from build123d import *

# Parameters (mm, degrees)
F3_DEPTH = 2.541


with BuildPart() as f1:
    # F0 (on Right) → F1 (revolve)
    with BuildSketch(Plane.YZ):
        with BuildLine():
            Line((16.51, 0), (19.05, 0))
            ThreePointArc((19.05, 0), (18.404048, 4.918689), (16.51, 9.50381))
            Line((16.51, 9.50381), (16.51, 0))
        make_face()
    revolve(axis=Axis((0, 17.78, 0), (0, -1, 0)))

    # F2 (on face) → F3 (cut, through all)
    with BuildSketch(Plane.XZ.offset(-16.51)):
        with BuildLine():
            Line((1.016, -4.826), (1.527208, -7.465389))
            ThreePointArc((1.527208, -7.465389), (5.388154, -5.388154), (7.465389, -1.527208))
            Line((7.465389, -1.527208), (4.826, -1.016))
            Line((4.826, -1.016), (4.826, 0))
            Line((4.826, 0), (4.826, 1.016))
            Line((4.826, 1.016), (7.465389, 1.527208))
            ThreePointArc((7.465389, 1.527208), (5.388154, 5.388154), (1.527208, 7.465389))
            Line((1.527208, 7.465389), (1.016, 4.826))
            Line((1.016, 4.826), (0, 4.826))
            Line((0, 4.826), (-1.016, 4.826))
            Line((-1.016, 4.826), (-1.527208, 7.465389))
            ThreePointArc((-1.527208, 7.465389), (-5.388154, 5.388154), (-7.465389, 1.527208))
            Line((-7.465389, 1.527208), (-4.826, 1.016))
            Line((-4.826, 1.016), (-4.826, 0))
            Line((-4.826, 0), (-4.826, -1.016))
            Line((-4.826, -1.016), (-7.465389, -1.527208))
            ThreePointArc((-7.465389, -1.527208), (-5.388154, -5.388154), (-1.527208, -7.465389))
            Line((-1.527208, -7.465389), (-1.016, -4.826))
            Line((-1.016, -4.826), (0, -4.826))
            Line((0, -4.826), (1.016, -4.826))
        make_face()
    extrude(amount=-F3_DEPTH, mode=Mode.SUBTRACT)


solid = f1.part
Part model, mm, in its own coordinate system. Coordinates: 2 decimals unless noted, no trailing zeros.
(1) Pull direction Z, two halves, no side cores. Call faces 1 (the face through (-0.7, 16.51, -5)), 2 (the face through (0, 17, 4.826)): pulls with the +Z half, pulls with the -Z half, needs draft (parallel to the pull), parting line crosses it, or undercut.
Check sheet entries:
face 1: needs draft
face 2: undercut
(2) Slice it at A-A, the plane x = 6.5. State how many separate pieces and enclosed holes the cut face has, and give its area (3 significant figures).
Check sheet entries:
separate pieces: 3
enclosed holes: 0
area: 6.79 mm2
(3) Pin check, flat tips, straight feed: pin 1 Ø0.6 at (y, z) = (17, 0.5) entering from +X; pin 2 Ø0.6 at (y, z) = (17.5, 0) entering from -X; pin 3 Ø8 at (x, z) = (-2.5, -3.5) entering from +Y. Stop position of each tip, or through.
Check sheet entries:
pin 1: stops at x = 9.15
pin 2: stops at x = -8.19
pin 3: stops at y = 18.43
(4) Probe L1, parallel to X at y = 16.9, z = 5.25; L2, parallel to X at y = 16.85, z = 3; L3, parallel to X at y = 16.95, z = -4.25. List the from-to ranges inside material, lowest first.
Check sheet entries:
L1: x = -7.05 to -5.52, -1.1 to 1.1, 5.52 to 7.05
L2: x = -8.37 to -7, 7 to 8.37
L3: x = -7.59 to -6.32, 6.32 to 7.59
